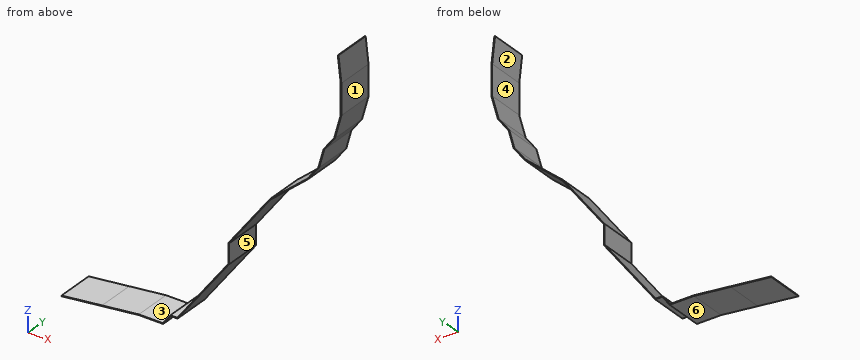
```python
from build123d import *

# Parameters (mm, degrees)
EXTRUDE_THIN1_START = -143.002
EXTRUDE_THIN1_DEPTH = 143.002
SKETCH2_W           = 353.476809532
SKETCH2_H           = 287.248033411
CUT_EXTRUDE1_DEPTH  = 2.54
SKETCH5_W           = 2.556683639
SKETCH5_H           = 143.002
BOSS_EXTRUDE1_DEPTH = 96.52
SKETCH6_W           = 436.207107494
SKETCH6_H           = 411.415497476
CUT_EXTRUDE3_DEPTH  = 2.54
SKETCH9_W           = 2.54
SKETCH9_H           = 143.002
BOSS_EXTRUDE2_DEPTH = 154.94


# Read off the part's stored shape, not the designer's step: Extrude-Thin1
with BuildPart() as part:
    # Extrude-Thin1 outline → Extrude-Thin1 (new body)
    with BuildSketch(Plane(origin=(0, 0, 0), x_dir=(1, 0, 0), z_dir=(0, 1, 0)).offset(EXTRUDE_THIN1_START)):
        Polygon((-482.832404898, 349.376524201), (-622.206225096, 365.37714102), (-602.245423716, 539.246259561), (-604.768848946, 539.535957871), (-625.019348636, 363.143414101), (-482.977728206, 346.836524201), (-392.100936643, 346.836524201), (-363.661203016, 308.759389966), (-337.521866174, 308.759389966), (-143.704865867, 49.263431443), (-143.704865867, -25.633038127), (14.14991429, -236.980223457), (156.541730962, -359.006376852), (198.09556878, -414.64160471), (217.458740987, -485.473629066), (257.724926693, -539.38485687), (282.185626339, -628.864042129), (282.185626339, -746.088969303), (429.494620494, -763.000572689), (429.784318804, -760.477147459), (284.725626339, -743.823886817), (284.725626339, -628.523119941), (260.048068344, -538.25064959), (219.781882638, -484.339421786), (200.418710431, -413.50739743), (158.408303922, -357.260882997), (16.016487249, -235.234729602), (-141.164865867, -24.789176199), (-141.164865867, 50.107293372), (-336.248708228, 311.299389966), (-362.38804507, 311.299389966), (-390.827778697, 349.376524201), align=None)
    extrude(amount=EXTRUDE_THIN1_DEPTH)

    # Sketch2 → Cut-Extrude1 (cut)
    with BuildSketch(Plane(origin=(-80.868694539, 0, 704.409024928), x_dir=(0.9934744998263692, 0, 0.11405445276158947), z_dir=(-0.11405445276158947, 0, 0.9934744998263692))):
        with Locations((435.779818352, -64.905243111)):
            Rectangle(SKETCH2_W, SKETCH2_H)
    extrude(amount=-CUT_EXTRUDE1_DEPTH, mode=Mode.SUBTRACT)

    # Sketch5 → Boss-Extrude1 (add)
    with BuildSketch(Plane(origin=(-80.578996229, 0, 701.885599699), x_dir=(0.9934744998263692, 0, 0.11405445276158968), z_dir=(-0.1140544527615897, 0, 0.9934744998263693))):
        with Locations((366.425733757, -71.501)):
            Rectangle(SKETCH5_W, SKETCH5_H)
    extrude(amount=BOSS_EXTRUDE1_DEPTH)

    # Sketch6 → Cut-Extrude3 (cut)
    with BuildSketch(Plane(origin=(-658.036684967, 0, -75.544982799), x_dir=(-0.11405445276159007, 0, 0.9934744998263692), z_dir=(-0.993474499826369, 0, -0.11405445276159006))):
        with Locations((-358.307764933, -83.68082163)):
            Rectangle(SKETCH6_W, SKETCH6_H)
    extrude(amount=-CUT_EXTRUDE3_DEPTH, mode=Mode.SUBTRACT)

    # Sketch9 → Boss-Extrude2 (add)
    with BuildSketch(Plane(origin=(-655.513259738, 0, -75.255284489), x_dir=(-0.11405445276159011, 0, 0.9934744998263692), z_dir=(-0.993474499826369, 0, -0.1140544527615901))):
        with Locations((-290.757481915, -71.501)):
            Rectangle(SKETCH9_W, SKETCH9_H)
    extrude(amount=BOSS_EXTRUDE2_DEPTH)


solid = part.part
```
Could you check a few things on this model? Use its own coordinates, in mm. Face numbers are marked on the shaded views. A direction names the side the tool comes from. Give positions to 0.01 mm unless a question says otherwise; leave off trailing zeros. Order: outer loops, then holes, each group sorted by start corner. A loop starts at its lowest first (then second) coordinate and runs counter-clockwise, first axis right, second up.
Q1. If I drill on line 1 along X through (y, z) = (-27, 8); line 2 along Z through (x, y) = (-474, -5.5); line 3 along X through (y, z) = (-35, 714), over which ranges is the centre line in solid material (lowest first)?
Q2. Suppose I cut it at B-B, the plane z = 682. Write out the boundary of the cut face in (x, y), and give its area (3 significant figures).
Q3. We'd pull the mould along Z, two halves only. Please class the marked faces 4, 5 and 6: +Z half, -Z half, draft (parallel to the pull), parting line (faces both ways), or undercut.
Q4. Suppose I cut it at C-C, the plane x = -97.5. Write out the boundary of the cut face in (y, z).
Q5. I'm going to push flat-ended pins straight in: P1, Ø6, axis at y = -64.5, z = -94, coming from the -X side; P2, Ø5, axis at y = -44.5, z = 572.5, coming from the +X side; P3, Ø13, axis at x = -351.5, y = -91.5, coming from the -Z side. Where does each tip first touch, or does it pass through?
Q6. For the marked faces 1, 2 and 3, which set-ups out of +Z, -Z, +X, -X, +Y, -Y let a thin tool reach every point of the face, with its end or its side?
Solution:
1. line 1: x = -143.7 to -141.16
1. line 2: z = -349.38 to -346.84
1. line 3: x = 282.19 to 284.73
2. outline: (282.19, -143) - (284.73, -143) - (284.73, 0) - (282.19, 0) - close
2. area: 363 mm2
3. face 4: undercut
3. face 5: draft
3. face 6: -Z half
4. outline: (-143, 83.25) - (0, 83.25) - (0, 87.5) - (-143, 87.5) - close
5. P1: stops at x = -179.36
5. P2: stops at x = 270.09
5. P3: stops at z = -311.3
6. face 1: +Z, -Z, +X, +Y, -Y
6. face 2: -X, +Y, -Y
6. face 3: +Z, -X, +Y, -Y
